Verification items for this drawing (mm, ordinates from the low corner). Round coordinates to 2 decimals unless told otherwise and drop trailing zeros. Order: outer loops, then holes, each group sorted by start corner. A loop starts at its lowest first (then second) coordinate and runs counter-clockwise, first axis right, second up.
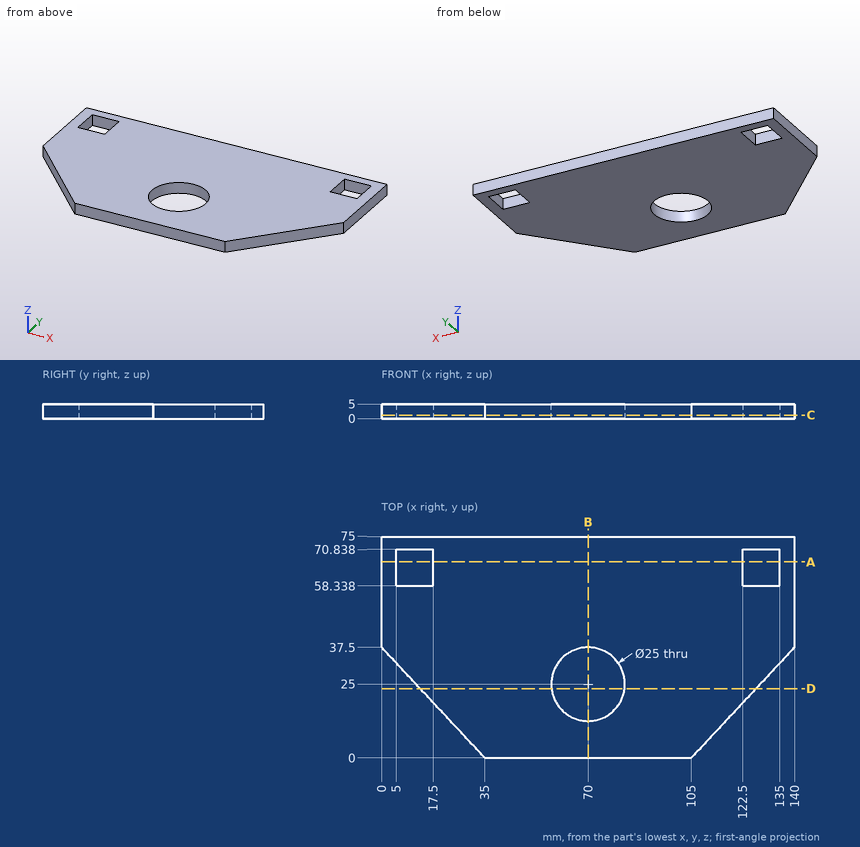
Item 1: Sectioned sample at D-D (y = 23.5). Record the cut outline in (x, z).
Answer:
outline: (13.07, 0) - (57.59, 0) - (57.59, 5) - (13.07, 5) - close; (82.41, 0) - (126.93, 0) - (126.93, 5) - (82.41, 5) - close
Item 2: Scan lines: line 1 along X through (y, z) = (61, 3.2); line 2 along Y through (x, z) = (70, 2); line 3 along Y through (x, z) = (134, 0.2). Record each from-to range of solid material in increasing order.
Answer:
line 1: x = 0 to 5, 17.5 to 122.5, 135 to 140
line 2: y = 0 to 12.5, 37.5 to 75
line 3: y = 31.07 to 58.34, 70.84 to 75
Item 3: Sectioned sample at A-A (y = 66.5). Record the cut outline in (x, z).
Answer:
outline: (0, 0) - (5, 0) - (5, 5) - (0, 5) - close; (17.5, 0) - (122.5, 0) - (122.5, 5) - (17.5, 5) - close; (135, 0) - (140, 0) - (140, 5) - (135, 5) - close
Item 4: Sectioned sample at C-C (z = 1.25). Record the cut outline in (x, y).
Answer:
outline: (0, 37.5) - (35, 0) - (105, 0) - (140, 37.5) - (140, 75) - (0, 75) - close; hole (5, 58.34) - (17.5, 58.34) - (17.5, 70.84) - (5, 70.84) - close; hole circle Ø25 at (70, 25); hole (122.5, 58.34) - (135, 58.34) - (135, 70.84) - (122.5, 70.84) - close
Item 5: Sectioned sample at B-B (x = 70). Record the cut outline in (y, z), and give its area (3 significant figures).
Answer:
outline: (0, 0) - (12.5, 0) - (12.5, 5) - (0, 5) - close; (37.5, 0) - (75, 0) - (75, 5) - (37.5, 5) - close
area: 250 mm2
Item 6: Go/stop test with a flat-tipped pin: P1, Ø2.5, axis at x = 131, z = 3, coming from the -Y side. Record where the tip stops, or that it passes through.
Answer:
P1: stops at y = 26.52
